CAD build for the part. Positions are in the model's coordinates, mm. A direction names the side the tool comes from. Give positions to 0.01 mm unless a question says otherwise; leave off trailing zeros. Order: outer loops, then holes, each group sorted by start corner. A loop starts at its lowest first (then second) coordinate and runs counter-clockwise, first axis right, second up. Notation, with made-up numbers: M -29.75,-10.5 L 13.25,-10.5 A25 ccw 13.25,19.5 Z; hole C 32,73.5 d4. An arc over 180 degrees is marked long. Put each result on its own line as item: value. Start each with the question number.
1) Drill centre lines: line 1 (Z direction, x = 0, y = -36.35); line 2 (Z direction, x = 24, y = -28); line 3 (X direction, y = -23, z = 1.25). Where is each one in solid material? Low to high. Write a range as [from, to].
2) Cut at C-C (x = 11). Write the cut outline in (y, z).
3) Cut at A-A (x = 24.2). Write the cut outline in (y, z).
4) Cut at B-B (z = -5). Write the cut outline in (x, y), and give its area (3 significant figures).
5) Pin check, flat tips, straight feed: pin 1 (5 mm diameter, centred on y = -20, z = -5, fed in from +X); pin 2 (1 mm diameter, centred on x = -6, z = 0.5, fed in from -Y); pin 3 (4 mm diameter, centred on x = -24.2, z = 5, fed in from +Y); pin 4 (0.8 mm diameter, centred on x = -25.5, z = 0, fed in from -Y). Stop position of each tip, or through.
6) Cut at D-D (y = -30). Write the cut outline in (x, z).
7) Two-plate mould, pull along X, no slides. Class faces 6 (the face through (-24, -31, 0.75)), 7 (the face through (-23.017, -27.732, 6.855)), 8 (the face through (-0.54, -36.51, -2.44)), 9 (the face through (27, -28, 0)): released by +X, released by -X, zero draft, split by the parting line, or undercut.
8) Tool access for faces 1 (the face through (13.54, -40.45, -1.05)), 2 (the face through (24, -31, -0.75)), 3 (the face through (24, -26.5, 0)), 4 (the face through (-22, -29, -6)), 5 (the face through (24, -32.4, 0)): list every direction of +Z, -Z, +X, -X, +Y, -Y with a clear straight run to the whole face (end or side of a thin tool).
```python
from build123d import *

# Parameters (mm, degrees)
F0_W      = 41
F0_H      = 20
F1_DEPTH  = 26.5
F2_W      = 6.5
F2_H      = 20
F2_R      = 2.2
F2_W_2    = 41
F3_DEPTH  = 2.5
F4_W      = 41
F4_H      = 20
F5_DEPTH  = 8
F6_W      = 6.5
F6_H      = 1.5
F7_DEPTH  = 3.4
F8_R      = 2.75
F9_DEPTH  = 7
F10_R     = 3
F10_R_2   = 2.5
F11_DEPTH = 1


# Not quite as in the source:
# - a pattern or mirror of a feature is missing from the dataset's text; its kind, count and spacing are read off the source's solid


with BuildPart() as f1:
    # F0 (on Front) → F1 (new body)
    with BuildSketch(Plane.XZ):
        Rectangle(F0_W, F0_H)
    extrude(amount=F1_DEPTH)

    # F2 (on face) → F3 (join)
    with BuildSketch(Plane.XZ.offset(26.5)):
        with Locations((-23.75, 0)):
            Rectangle(F2_W, F2_H)
        with Locations((-24.2, -5)):
            Circle(F2_R, mode=Mode.SUBTRACT)
        with Locations((-24.2, 5)):
            Circle(F2_R, mode=Mode.SUBTRACT)
        with Locations((23.75, 0)):
            Rectangle(F2_W, F2_H)
        with Locations((24.2, -5)):
            Circle(F2_R, mode=Mode.SUBTRACT)
        with Locations((24.2, 5)):
            Circle(F2_R, mode=Mode.SUBTRACT)
        Rectangle(F2_W_2, F2_H)
    extrude(amount=F3_DEPTH)

    # F4 (on face) → F5 (join)
    with BuildSketch(Plane.XZ.offset(29)):
        Rectangle(F4_W, F4_H)
    extrude(amount=F5_DEPTH)

    # F6 (on face) → F7 (join)
    with BuildSketch(Plane.XZ.offset(29)):
        with Locations((-23.75, 0)):
            Rectangle(F6_W, F6_H)
    f7 = extrude(amount=F7_DEPTH)

    # F7_copies: F7 across plane
    add(f7.mirror(Plane(origin=(0, 0, 0), x_dir=(0, 0, 1), z_dir=(1, 0, 0))))

    # F8 (on face) → F9 (join)
    with BuildSketch(Plane.XZ.offset(37)):
        with Locations((11, 0)):
            Circle(F8_R)
    extrude(amount=F9_DEPTH)

    # F10 (on face) → F11 (cut)
    with BuildSketch(Plane.XZ.offset(37)):
        Circle(F10_R)
        Circle(F10_R_2, mode=Mode.SUBTRACT)
    extrude(amount=-F11_DEPTH, mode=Mode.SUBTRACT)


solid = f1.part
```
Solution:
1. line 1: [-10, -3], [-2.5, 2.5], [3, 10]
1. line 2: [-10, -7.19], [-2.81, 2.81], [7.19, 10]
1. line 3: [-20.5, 20.5]
2. outline: M -44,-2.75 L -37,-2.75 L -37,-10 L 0,-10 L 0,10 L -37,10 L -37,2.75 L -44,2.75 Z
3. outline: M -32.4,-0.75 L -29,-0.75 L -29,-2.8 L -26.5,-2.8 L -26.5,2.8 L -29,2.8 L -29,0.75 L -32.4,0.75 Z; M -29,-10 L -26.5,-10 L -26.5,-7.2 L -29,-7.2 Z; M -29,7.2 L -26.5,7.2 L -26.5,10 L -29,10 Z
4. outline: M -27,-29 L -26.4,-29 L -26.4,-26.5 L -27,-26.5 Z; M -22,-29 L -20.5,-29 L -20.5,-37 L 20.5,-37 L 20.5,-29 L 22,-29 L 22,-26.5 L 20.5,-26.5 L 20.5,0 L -20.5,0 L -20.5,-26.5 L -22,-26.5 Z; M 26.4,-29 L 27,-29 L 27,-26.5 L 26.4,-26.5 Z
4. area: 1,530 mm²
5. pin 1: x = 20.5
5. pin 2: y = -37
5. pin 3: through
5. pin 4: y = -32.4
6. outline: M -27,-0.75 L -20.5,-0.75 L -20.5,-10 L 20.5,-10 L 20.5,-0.75 L 27,-0.75 L 27,0.75 L 20.5,0.75 L 20.5,10 L -20.5,10 L -20.5,0.75 L -27,0.75 Z
7. face 6: zero draft
7. face 7: undercut
7. face 8: undercut
7. face 9: released by +X
8. face 1: -Y
8. face 2: -Z, +X, -Y
8. face 3: +Z, -Z, +X, +Y
8. face 4: -Z, -X, -Y
8. face 5: +Z, -Z, +X, -Y
